Study the drawing (mm; zero at the part's minimum x, y, z) and answer. Coordinates: 2 decimals unless noted, no trailing zeros. Order: outer loops, then holes, each group sorted by start corner. A loop starts at its lowest first (then second) coordinate and runs counter-clockwise, first axis right, second up. Notation, with made-up numbers: M 84,65 L 129,65 A12 ccw 129,73 Z; hole C -23,10 d2. An arc over 180 degrees is marked long. One line per item, written item: value. Start each with the question number.
Q1. The part is cut by section A-A on y = 0.7. Give the vertices of the cut face in (x, z).
Q2. Straight lines are drawn through the part: line 1 along X through (y, z) = (0.2, 13); line 2 along Z through (x, y) = (59.5, 0.8) (1 decimal); line 3 along Z through (x, y) = (73.5, 0.4) (1 decimal). For each, find the intervals that lie inside material, in ascending order. Write a range as [from, to].
Q3. The part is cut by section C-C on z = 10.5. Give the vertices of the cut face in (x, y).
Q4. The part is cut by section B-B on x = 66. Give the vertices of the cut face in (y, z).
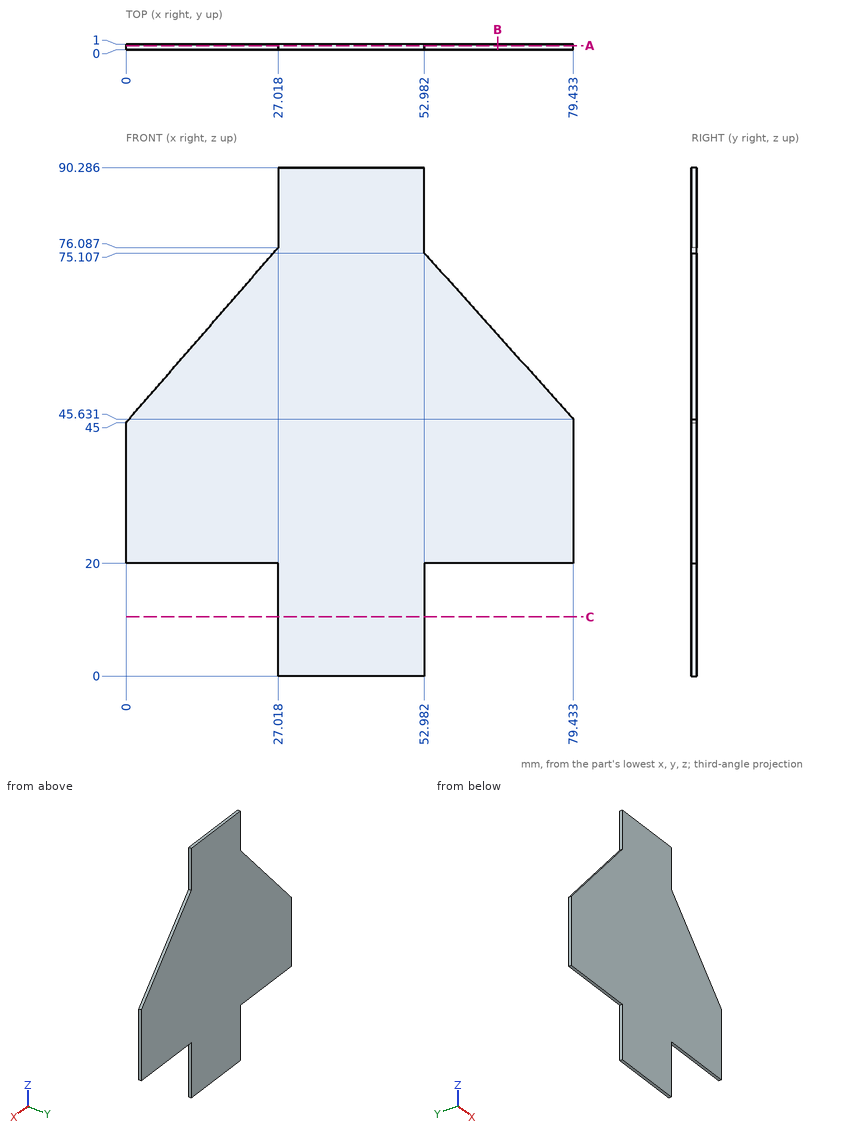
Output:
1. outline: M 0,20 L 27.02,20 L 27.02,0 L 52.98,0 L 52.98,20 L 79.43,20 L 79.43,45.63 L 52.98,75.11 L 52.98,90.29 L 27.02,90.29 L 27.02,76.09 L 0,45 Z
2. line 1: x = [27.02, 52.98]
2. line 2: z = [20, 67.8]
2. line 3: z = [20, 52.2]
3. outline: M 27.02,0 L 52.98,0 L 52.98,1 L 27.02,1 Z
4. outline: M 0,20 L 1,20 L 1,60.6 L 0,60.6 Z
